from build123d import *

# Parameters (mm, degrees)
SKETCH1_R           = 1.5
BOSS_EXTRUDE1_DEPTH = 3
SKETCH2_R           = 1.6
SKETCH2_R_2         = 1.5
BOSS_EXTRUDE2_DEPTH = 3
SKETCH3_R           = 5.25
SKETCH3_R_2         = 2.75
BOSS_EXTRUDE3_DEPTH = 5.5
CUT_EXTRUDE1_START  = -2
SKETCH4_R           = 2.75
CUT_EXTRUDE1_DEPTH  = 2


with BuildPart() as part:
    # Sketch1 → Boss-Extrude1 (new body)
    with BuildSketch(Plane(origin=(3, 0, 0), x_dir=(0, 0, -1), z_dir=(1, 0, 0))):
        with BuildLine():
            ThreePointArc((-14.537314892, 1.599093719), (-13.375367565, 0.916420874), (-12.080565177, 0.542722358))
            ThreePointArc((-12.080565177, 0.542722358), (-12.09275, 0), (-12.080565177, -0.542722358))
            ThreePointArc((-12.080565177, -0.542722358), (-13.375367565, -0.916420874), (-14.537314892, -1.599093719))
            ThreePointArc((-14.537314892, -1.599093719), (-14.499881098, -1.908945561), (-14.455843809, -2.217928037))
            ThreePointArc((-14.455843809, -2.217928037), (-13.156800143, -2.576605271), (-11.809396783, -2.602450802))
            ThreePointArc((-11.809396783, -2.602450802), (-11.680699536, -3.129834008), (-11.528463019, -3.650909885))
            ThreePointArc((-11.528463019, -3.650909885), (-12.682425791, -4.346994451), (-13.62809199, -5.30713988))
            ThreePointArc((-13.62809199, -5.30713988), (-13.511738163, -5.596745198), (-13.389230859, -5.883801663))
            ThreePointArc((-13.389230859, -5.883801663), (-12.041618533, -5.894040025), (-10.733437515, -5.57027124))
            ThreePointArc((-10.733437515, -5.57027124), (-10.472628702, -6.046375), (-10.190715157, -6.510293938))
            ThreePointArc((-10.190715157, -6.510293938), (-11.125197659, -7.48132754), (-11.79013714, -8.65351323))
            ThreePointArc((-11.79013714, -8.65351323), (-11.602792602, -8.903135899), (-11.410163953, -9.148703928))
            ThreePointArc((-11.410163953, -9.148703928), (-10.105820521, -8.809805691), (-8.926012217, -8.158486898))
            ThreePointArc((-8.926012217, -8.158486898), (-8.550865528, -8.550865528), (-8.158486898, -8.926012217))
            ThreePointArc((-8.158486898, -8.926012217), (-8.809805691, -10.105820521), (-9.148703928, -11.410163953))
            ThreePointArc((-9.148703928, -11.410163953), (-8.903135899, -11.602792602), (-8.65351323, -11.79013714))
            ThreePointArc((-8.65351323, -11.79013714), (-7.48132754, -11.125197659), (-6.510293938, -10.190715157))
            ThreePointArc((-6.510293938, -10.190715157), (-6.046375, -10.472628702), (-5.57027124, -10.733437515))
            ThreePointArc((-5.57027124, -10.733437515), (-5.894040025, -12.041618533), (-5.883801663, -13.389230859))
            ThreePointArc((-5.883801663, -13.389230859), (-5.596745198, -13.511738163), (-5.30713988, -13.62809199))
            ThreePointArc((-5.30713988, -13.62809199), (-4.346994451, -12.682425791), (-3.650909885, -11.528463019))
            ThreePointArc((-3.650909885, -11.528463019), (-3.129834008, -11.680699536), (-2.602450802, -11.809396783))
            ThreePointArc((-2.602450802, -11.809396783), (-2.576605271, -13.156800143), (-2.217928037, -14.455843809))
            ThreePointArc((-2.217928037, -14.455843809), (-1.908945561, -14.499881098), (-1.599093719, -14.537314892))
            ThreePointArc((-1.599093719, -14.537314892), (-0.916420874, -13.375367565), (-0.542722358, -12.080565177))
            ThreePointArc((-0.542722358, -12.080565177), (0, -12.09275), (0.542722358, -12.080565177))
            ThreePointArc((0.542722358, -12.080565177), (0.916420874, -13.375367565), (1.599093719, -14.537314892))
            ThreePointArc((1.599093719, -14.537314892), (1.908945561, -14.499881098), (2.217928037, -14.455843809))
            ThreePointArc((2.217928037, -14.455843809), (2.576605271, -13.156800143), (2.602450802, -11.809396783))
            ThreePointArc((2.602450802, -11.809396783), (3.129834008, -11.680699536), (3.650909885, -11.528463019))
            ThreePointArc((3.650909885, -11.528463019), (4.346994451, -12.682425791), (5.30713988, -13.62809199))
            ThreePointArc((5.30713988, -13.62809199), (5.596745198, -13.511738163), (5.883801663, -13.389230859))
            ThreePointArc((5.883801663, -13.389230859), (5.894040025, -12.041618533), (5.57027124, -10.733437515))
            ThreePointArc((5.57027124, -10.733437515), (6.046375, -10.472628702), (6.510293938, -10.190715157))
            ThreePointArc((6.510293938, -10.190715157), (7.48132754, -11.125197659), (8.65351323, -11.79013714))
            ThreePointArc((8.65351323, -11.79013714), (8.903135899, -11.602792602), (9.148703928, -11.410163953))
            ThreePointArc((9.148703928, -11.410163953), (8.809805691, -10.105820521), (8.158486898, -8.926012217))
            ThreePointArc((8.158486898, -8.926012217), (8.550865528, -8.550865528), (8.926012217, -8.158486898))
            ThreePointArc((8.926012217, -8.158486898), (10.105820521, -8.809805691), (11.410163953, -9.148703928))
            ThreePointArc((11.410163953, -9.148703928), (11.602792602, -8.903135899), (11.79013714, -8.65351323))
            ThreePointArc((11.79013714, -8.65351323), (11.125197659, -7.48132754), (10.190715157, -6.510293938))
            ThreePointArc((10.190715157, -6.510293938), (10.472628702, -6.046375), (10.733437515, -5.57027124))
            ThreePointArc((10.733437515, -5.57027124), (12.041618533, -5.894040025), (13.389230859, -5.883801663))
            ThreePointArc((13.389230859, -5.883801663), (13.511738163, -5.596745198), (13.62809199, -5.30713988))
            ThreePointArc((13.62809199, -5.30713988), (12.682425791, -4.346994451), (11.528463019, -3.650909885))
            ThreePointArc((11.528463019, -3.650909885), (11.680699536, -3.129834008), (11.809396783, -2.602450802))
            ThreePointArc((11.809396783, -2.602450802), (13.156800143, -2.576605271), (14.455843809, -2.217928037))
            ThreePointArc((14.455843809, -2.217928037), (14.499881098, -1.908945561), (14.537314892, -1.599093719))
            ThreePointArc((14.537314892, -1.599093719), (13.375367565, -0.916420874), (12.080565177, -0.542722358))
            ThreePointArc((12.080565177, -0.542722358), (12.09275, 0), (12.080565177, 0.542722358))
            ThreePointArc((12.080565177, 0.542722358), (13.375367565, 0.916420874), (14.537314892, 1.599093719))
            ThreePointArc((14.537314892, 1.599093719), (14.499881098, 1.908945561), (14.455843809, 2.217928037))
            ThreePointArc((14.455843809, 2.217928037), (13.156800143, 2.576605271), (11.809396783, 2.602450802))
            ThreePointArc((11.809396783, 2.602450802), (11.680699536, 3.129834008), (11.528463019, 3.650909885))
            ThreePointArc((11.528463019, 3.650909885), (12.682425791, 4.346994451), (13.62809199, 5.30713988))
            ThreePointArc((13.62809199, 5.30713988), (13.511738163, 5.596745198), (13.389230859, 5.883801663))
            ThreePointArc((13.389230859, 5.883801663), (12.041618533, 5.894040025), (10.733437515, 5.57027124))
            ThreePointArc((10.733437515, 5.57027124), (10.472628702, 6.046375), (10.190715157, 6.510293938))
            ThreePointArc((10.190715157, 6.510293938), (11.125197659, 7.48132754), (11.79013714, 8.65351323))
            ThreePointArc((11.79013714, 8.65351323), (11.602792602, 8.903135899), (11.410163953, 9.148703928))
            ThreePointArc((11.410163953, 9.148703928), (10.105820521, 8.809805691), (8.926012217, 8.158486898))
            ThreePointArc((8.926012217, 8.158486898), (8.550865528, 8.550865528), (8.158486898, 8.926012217))
            ThreePointArc((8.158486898, 8.926012217), (8.809805691, 10.105820521), (9.148703928, 11.410163953))
            ThreePointArc((9.148703928, 11.410163953), (8.903135899, 11.602792602), (8.65351323, 11.79013714))
            ThreePointArc((8.65351323, 11.79013714), (7.48132754, 11.125197659), (6.510293938, 10.190715157))
            ThreePointArc((6.510293938, 10.190715157), (6.046375, 10.472628702), (5.57027124, 10.733437515))
            ThreePointArc((5.57027124, 10.733437515), (5.894040025, 12.041618533), (5.883801663, 13.389230859))
            ThreePointArc((5.883801663, 13.389230859), (5.596745198, 13.511738163), (5.30713988, 13.62809199))
            ThreePointArc((5.30713988, 13.62809199), (4.346994451, 12.682425791), (3.650909885, 11.528463019))
            ThreePointArc((3.650909885, 11.528463019), (3.129834008, 11.680699536), (2.602450802, 11.809396783))
            ThreePointArc((2.602450802, 11.809396783), (2.576605271, 13.156800143), (2.217928037, 14.455843809))
            ThreePointArc((2.217928037, 14.455843809), (1.908945561, 14.499881098), (1.599093719, 14.537314892))
            ThreePointArc((1.599093719, 14.537314892), (0.916420874, 13.375367565), (0.542722358, 12.080565177))
            ThreePointArc((0.542722358, 12.080565177), (0, 12.09275), (-0.542722358, 12.080565177))
            ThreePointArc((-0.542722358, 12.080565177), (-0.916420874, 13.375367565), (-1.599093719, 14.537314892))
            ThreePointArc((-1.599093719, 14.537314892), (-1.908945561, 14.499881098), (-2.217928037, 14.455843809))
            ThreePointArc((-2.217928037, 14.455843809), (-2.576605271, 13.156800143), (-2.602450802, 11.809396783))
            ThreePointArc((-2.602450802, 11.809396783), (-3.129834008, 11.680699536), (-3.650909885, 11.528463019))
            ThreePointArc((-3.650909885, 11.528463019), (-4.346994451, 12.682425791), (-5.30713988, 13.62809199))
            ThreePointArc((-5.30713988, 13.62809199), (-5.596745198, 13.511738163), (-5.883801663, 13.389230859))
            ThreePointArc((-5.883801663, 13.389230859), (-5.894040025, 12.041618533), (-5.57027124, 10.733437515))
            ThreePointArc((-5.57027124, 10.733437515), (-6.046375, 10.472628702), (-6.510293938, 10.190715157))
            ThreePointArc((-6.510293938, 10.190715157), (-7.48132754, 11.125197659), (-8.65351323, 11.79013714))
            ThreePointArc((-8.65351323, 11.79013714), (-8.903135899, 11.602792602), (-9.148703928, 11.410163953))
            ThreePointArc((-9.148703928, 11.410163953), (-8.809805691, 10.105820521), (-8.158486898, 8.926012217))
            ThreePointArc((-8.158486898, 8.926012217), (-8.550865528, 8.550865528), (-8.926012217, 8.158486898))
            ThreePointArc((-8.926012217, 8.158486898), (-10.105820521, 8.809805691), (-11.410163953, 9.148703928))
            ThreePointArc((-11.410163953, 9.148703928), (-11.602792602, 8.903135899), (-11.79013714, 8.65351323))
            ThreePointArc((-11.79013714, 8.65351323), (-11.125197659, 7.48132754), (-10.190715157, 6.510293938))
            ThreePointArc((-10.190715157, 6.510293938), (-10.472628702, 6.046375), (-10.733437515, 5.57027124))
            ThreePointArc((-10.733437515, 5.57027124), (-12.041618533, 5.894040025), (-13.389230859, 5.883801663))
            ThreePointArc((-13.389230859, 5.883801663), (-13.511738163, 5.596745198), (-13.62809199, 5.30713988))
            ThreePointArc((-13.62809199, 5.30713988), (-12.682425791, 4.346994451), (-11.528463019, 3.650909885))
            ThreePointArc((-11.528463019, 3.650909885), (-11.680699536, 3.129834008), (-11.809396783, 2.602450802))
            ThreePointArc((-11.809396783, 2.602450802), (-13.156800143, 2.576605271), (-14.455843809, 2.217928037))
            ThreePointArc((-14.455843809, 2.217928037), (-14.499881098, 1.908945561), (-14.537314892, 1.599093719))
        make_face()
        with Locations(Location((0, 0, 0), (0, 0, 180))):
            Circle(SKETCH1_R, mode=Mode.SUBTRACT)
    extrude(amount=-BOSS_EXTRUDE1_DEPTH)

    # Sketch2 → Boss-Extrude2 (add)
    with BuildSketch(Plane(origin=(3, 0, 0), x_dir=(0, 0, -1), z_dir=(1, 0, 0))):
        with BuildLine():
            Line((0.522104769, -3.965779445), (-44.092913993, -9.839458095))
            ThreePointArc((-44.092913993, -9.839458095), (-48.580798207, -6.395783419), (-45.137123531, -1.907899204))
            Line((-45.137123531, -1.907899204), (-0.522104769, 3.965779445))
            ThreePointArc((-0.522104769, 3.965779445), (3.965779445, 0.522104769), (0.522104769, -3.965779445))
        make_face()
        with Locations((-44.615018762, -5.87367865)):
            Circle(SKETCH2_R, mode=Mode.SUBTRACT)
        with Locations(Location((0, 0, 0), (0, 0, 180))):
            Circle(SKETCH2_R_2, mode=Mode.SUBTRACT)
    extrude(amount=-BOSS_EXTRUDE2_DEPTH)

    # Sketch3 → Boss-Extrude3 (add)
    with BuildSketch(Plane(origin=(3, 0, 0), x_dir=(0, 0, -1), z_dir=(1, 0, 0))):
        Circle(SKETCH3_R)
        Circle(SKETCH3_R_2, mode=Mode.SUBTRACT)
    extrude(amount=BOSS_EXTRUDE3_DEPTH)

    # Sketch4 → Cut-Extrude1 (cut)
    with BuildSketch(Plane(origin=(3, 0, 0), x_dir=(0, 0, -1), z_dir=(1, 0, 0)).offset(CUT_EXTRUDE1_START)):
        Circle(SKETCH4_R)
    extrude(amount=CUT_EXTRUDE1_DEPTH, mode=Mode.SUBTRACT)


solid = part.part
Here's how the part is built. I have some questions about the finished solid (model axes, mm). A direction names the side the tool comes from. Coordinates: 2 decimals unless noted, no trailing zeros. Loops run counter-clockwise (first coordinate to the right, second up) from the corner with the lowest first, then second, coordinate; pieces in that order, holes last.
1. I need wall thicknesses on L1, parallel to Y at x = 0.35, z = 0; L2, parallel to Z at x = 2.25, y = -10.75; L3, parallel to Z at x = 1.5, y = 12. Which ranges of each line are inside material? Lowest first, please.
2. Imagine slicing it at C-C, the plane y = 7.5. Please give me the cut outline in (x, z).
3. For faces 4 (the cylindrical face through (1.52, 4.36, 12.7)), 5 (the cylindrical face through (1.521, 2.574, -13.176)), 6 (the cylindrical face through (1.521, -0.924, -13.393)), 7 (the cylindrical face through (1.52, 11.14, -7.5)), which set-ups out of +Z, -Z, +X, -X, +Y, -Y let a thin tool reach every point of the face, with its end or its side?
4. Imagine slicing it at B-B, the plane z = 20. Please give me the cut outline in (x, y), and give its area (3 significant figures).
5. If we mould it in two halves opening along Y, with no side actions, what happens to faces 1 (the cylindrical face through (5.7, 1.6, -5)), 2 (the cylindrical face through (1.521, 12.668, 4.335)), 3 (the cylindrical face through (1.52, 7.5, 11.14))? For each: pulls with the +Y half, pulls with the -Y half, needs draft (parallel to the pull), parting line crosses it, or undercut.
6. Imagine slicing it at A-A, the plane x = 4. Please give me the cut outline in (y, z).
7. For P1, Ø4.5, axis at y = 0, z = 0, coming from the -X side; P2, Ø5, axis at x = 3, z = 17, coming from the +Y side; P3, Ø1.5, axis at x = 5, y = 10, coming from the +Z side; P4, Ø4, axis at x = 3, z = 24, coming from the -Y side, each with a flat end and sliding along its axis, tell me the tip position at first contact or that it passes through.
Taken from the geometry:
1. L1: y = -12.09 to -1.5, 1.5 to 12.09
1. L2: z = -9.02 to -7.03, -5.58 to 5.58, 7.03 to 9.02
1. L3: z = -5.89 to -3.89, -2.62 to 2.62, 3.89 to 5.89
2. outline: (0, -11.14) - (3, -11.14) - (3, 11.14) - (0, 11.14) - close
3. face 4: +Z, +X, -X
3. face 5: +X, -X
3. face 6: -Z, +X, -X
3. face 7: +X, -X, +Y
4. outline: (0, -6.67) - (3, -6.67) - (3, 1.4) - (0, 1.4) - close
4. area: 24.2 mm2
5. face 1: parting line crosses it
5. face 2: pulls with the +Y half
5. face 3: undercut
6. outline: circle Ø10.5 at (0, 0); hole circle Ø5.5 at (0, 0)
7. P1: stops at x = 0
7. P2: stops at y = 2.13
7. P3: passes through
7. P4: stops at y = -7.46
